Autodesk Inventor part; units mm, degrees
ref_plane "YZ Plane" through (0, 0, 0) normal (1, 0, 0) x (0, 1, 0)
ref_plane "XZ Plane" through (0, 0, 0) normal (0, 1, 0) x (-1, 0, 0)
ref_plane "XY Plane" through (0, 0, 0) normal (0, 0, 1) x (1, 0, 0)
sketch "Sketch1" plane through (0, 0, 0) normal (0, 0, 1) x (1, 0, 0)
  line L0 (49.8602, 49.276) -> (49.8602, -49.276)
  line L1 (49.8602, -49.276) -> (-49.7078, -49.276)
  line L2 (-49.7078, -49.276) -> (-49.7078, 49.276)
  line L3 (49.8602, 49.276) -> (16.0782, 49.276)
  line L4 (16.0782, 49.276) -> (16.0782, 39.116)
  line L5 (16.0782, 39.116) -> (-15.9258, 39.116)
  line L6 (-15.9258, 39.116) -> (-15.9258, 49.276)
  line L7 (-49.7078, 49.276) -> (-15.9258, 49.276)
  line L8 (16.0782, 49.276) -> (49.8602, 49.276)
  line L9 (-46.5164, 37.846) -> (-41.7666, 37.846)
  line L10 (-41.7666, 37.846) -> (-41.7666, 27.813)
  line L11 (-41.7666, 27.813) -> (-46.5164, 27.813)
  line L12 (-46.5164, 27.813) -> (-46.5164, 37.846)
  line L13 (42.037, 37.846) -> (46.7868, 37.846)
  line L14 (46.7868, 37.846) -> (46.7868, 27.813)
  line L15 (46.7868, 27.813) -> (42.037, 27.813)
  line L16 (42.037, 27.813) -> (42.037, 37.846)
  line L17 (-46.5926, -43.2793) -> (-46.5926, -46.0733)
  line L18 (-46.5926, -43.2793) -> (-38.4646, -43.2793)
  line L19 (-38.4646, -43.2793) -> (-38.4646, -46.0733)
  line L20 (-38.4646, -46.0733) -> (-46.5926, -46.0733)
  line L21 (46.5926, -43.2793) -> (38.4646, -43.2793)
  line L22 (38.4646, -43.2793) -> (38.4646, -46.0733)
  line L23 (38.4646, -46.0733) -> (46.5926, -46.0733)
  line L24 (46.5926, -43.2793) -> (46.5926, -46.0733)
  point P0 (0, 0)
  dimension "d0" = 99.568
  dimension "d1" = 98.552
  dimension "d2" = 33.782
  dimension "d3" = 10.16
  dimension "d4" = 32.004
  dimension "d9" = 4.7498
  dimension "d10" = 10.033
  dimension "d12" = 3.1914
  dimension "d13" = 4.7498
  dimension "d14" = 10.033
  dimension "d23" = 8.128
  dimension "d25" = 2.794
extrude "Extrusion3" add sketch "Sketch1" along normal blind 2.54
properties part number "RTS Frame Front Panel"
Read the model definition and answer for the solid it produces. Units are mm, in the model's axes. A direction names the side the tool comes from. Coordinates: 2 decimals unless noted, no trailing zeros. Loops run counter-clockwise (first coordinate to the right, second up) from the corner with the lowest first, then second, coordinate; pieces in that order, holes last.
Q1. Consider probe 1 along Y at (x, z) = (-45, 0.35); probe 2 along X at (y, z) = (31, 2.1); probe 3 along Y at (x, z) = (-39.5, 2.15). Determine where each line is inside the solid, lowest interval first.
Q2. This flat-tipped pin is pushed along its axis until it touches: pin 1 Ø0.8 at (x, z) = (-6.5, 1) entering from +Y. Where does it stop, or does it pass through?
Q3. Which of the six approach directions +Z, -Z, +X, -X, +Y, -Y give full straight-line access (tool end or side, diameter ignored) to faces 4 (the face through (-42, -46.073, 1)), 5 (the face through (-33, 49.276, 1)), 6 (the face through (16.078, 44, 1))?
Q4. The part is cut by section C-C on x = -6. Write down the section's boundary in (y, z), and give its area (3 significant figures).
Q5. The part is cut by section B-B on y = 32. Write down the section's boundary in (x, z), and give its area (3 significant figures).
Q6. The mould has two halves that part along X. Classify faces 1 (the face through (33, 49.276, 1)), 2 (the face through (49.86, 1, 1)), 3 (the face through (0, 39.116, 1)): +X half, -X half, draft (parallel to the pull), parting line (faces both ways), or undercut.
Q7. The part is cut by section A-A on z = 2.1. Write down the section's boundary in (x, y), and give its area (3 significant figures).
Results below:
1. probe 1: y = -49.28 to -46.07, -43.28 to 27.81, 37.85 to 49.28
1. probe 2: x = -49.71 to -46.52, -41.77 to 42.04, 46.79 to 49.86
1. probe 3: y = -49.28 to -46.07, -43.28 to 49.28
2. pin 1: stops at y = 39.12
3. face 4: +Z, -Z
3. face 5: +Z, -Z, +X, -X, +Y
3. face 6: +Z, -Z, +Y
4. outline: (-49.28, 0) - (39.12, 0) - (39.12, 2.54) - (-49.28, 2.54) - close
4. area: 225 mm2
5. outline: (-49.71, 0) - (-46.52, 0) - (-46.52, 2.54) - (-49.71, 2.54) - close; (-41.77, 0) - (42.04, 0) - (42.04, 2.54) - (-41.77, 2.54) - close; (46.79, 0) - (49.86, 0) - (49.86, 2.54) - (46.79, 2.54) - close
5. area: 229 mm2
6. face 1: draft
6. face 2: +X half
6. face 3: undercut
7. outline: (-49.71, -49.28) - (49.86, -49.28) - (49.86, 49.28) - (16.08, 49.28) - (16.08, 39.12) - (-15.93, 39.12) - (-15.93, 49.28) - (-49.71, 49.28) - close; hole (-46.59, -46.07) - (-38.46, -46.07) - (-38.46, -43.28) - (-46.59, -43.28) - close; hole (-46.52, 27.81) - (-41.77, 27.81) - (-41.77, 37.85) - (-46.52, 37.85) - close; hole (38.46, -46.07) - (46.59, -46.07) - (46.59, -43.28) - (38.46, -43.28) - close; hole (42.04, 27.81) - (46.79, 27.81) - (46.79, 37.85) - (42.04, 37.85) - close
7. area: 9,350 mm2
